from build123d import *

# Parameters (mm, degrees)
F1_DEPTH       = 6.35
F2_R           = 3.81
F3_DEPTH       = 6.35
F5_D           = 2.032
F5_CSINK_D     = 3.175
F5_CSINK_ANGLE = 82
F6_D           = 2.032
F6_CSINK_D     = 3.175
F6_CSINK_ANGLE = 82
F7_SIZE        = 0.508


with BuildPart() as f1:
    # F0 (on Right) → F1 (new body)
    with BuildSketch(Plane.YZ):
        with BuildLine():
            ThreePointArc((-5.08, 12.7), (-3.5921024484, 9.1078975516), (0, 7.62))
            Line((0, 7.62), (0, 12.7))
            Line((0, 12.7), (0, 17.78))
            ThreePointArc((0, 17.78), (-3.5921024484, 16.2921024484), (-5.08, 12.7))
        make_face()
        with BuildLine():
            Line((0, 12.7), (0, 7.62))
            ThreePointArc((0, 7.62), (3.5921024484, 9.1078975516), (5.08, 12.7))
            ThreePointArc((5.08, 12.7), (3.5921024484, 16.2921024484), (0, 17.78))
            Line((0, 17.78), (0, 12.7))
        make_face()
        with BuildLine():
            ThreePointArc((5.08, 12.7), (3.5921024484, 9.1078975516), (0, 7.62))
            ThreePointArc((0, 7.62), (-3.5921024484, 9.1078975516), (-5.08, 12.7))
            Line((-5.08, 12.7), (-5.08, 0))
            ThreePointArc((-5.08, 0), (0, -5.08), (5.08, 0))
            Line((5.08, 0), (5.08, 12.7))
        make_face()
        with BuildLine():
            ThreePointArc((0, 17.78), (3.5921024484, 16.2921024484), (5.08, 12.7))
            Line((5.08, 12.7), (5.08, 32.7368881382))
            Line((5.08, 32.7368881382), (4.2115108686, 31.4493000504))
            ThreePointArc((4.2115108686, 31.4493000504), (2.384915539, 29.8046262283), (0, 29.21))
            Line((0, 29.21), (0, 17.78))
        make_face()
        with BuildLine():
            Line((-5.08, 34.29), (-5.08, 12.7))
            ThreePointArc((-5.08, 12.7), (-3.5921024484, 16.2921024484), (0, 17.78))
            Line((0, 17.78), (0, 29.21))
            ThreePointArc((0, 29.21), (-3.5921024484, 30.6978975516), (-5.08, 34.29))
        make_face()
        with BuildLine():
            Line((4.2115108686, 31.4493000504), (5.08, 32.7368881382))
            Line((5.08, 32.7368881382), (5.08, 34.29))
            ThreePointArc((5.08, 34.29), (4.4853737717, 36.674915539), (2.8406999496, 38.5015108686))
            Line((2.8406999496, 38.5015108686), (0, 34.29))
            Line((0, 34.29), (0, 29.21))
            ThreePointArc((0, 29.21), (2.384915539, 29.8046262283), (4.2115108686, 31.4493000504))
        make_face()
        with BuildLine():
            Line((5.08, 34.29), (5.08, 32.7368881382))
            Line((5.08, 32.7368881382), (26.9371104656, 65.141386999))
            ThreePointArc((26.9371104656, 65.141386999), (25.5662995467, 72.1935978172), (18.5140887285, 70.8227868983))
            Line((18.5140887285, 70.8227868983), (-4.2115108686, 37.1306999496))
            ThreePointArc((-4.2115108686, 37.1306999496), (-0.9693096965, 39.2766660919), (2.8406999496, 38.5015108686))
            ThreePointArc((2.8406999496, 38.5015108686), (4.4853737717, 36.674915539), (5.08, 34.29))
        make_face()
        with BuildLine():
            ThreePointArc((-4.2115108686, 37.1306999496), (-4.8580281603, 35.77524826), (-5.08, 34.29))
            ThreePointArc((-5.08, 34.29), (-3.5921024484, 30.6978975516), (0, 29.21))
            Line((0, 29.21), (0, 34.29))
            Line((0, 34.29), (2.8406999496, 38.5015108686))
            ThreePointArc((2.8406999496, 38.5015108686), (-0.9693096965, 39.2766660919), (-4.2115108686, 37.1306999496))
        make_face()
    extrude(amount=F1_DEPTH)

    # F2 (on face) → F3 (join)
    with BuildSketch(Plane.YZ.offset(6.35)):
        with Locations((0, 12.7)):
            Circle(F2_R)
    extrude(amount=F3_DEPTH)

    # F5 (through all)
    with Locations(Plane.YZ.offset(12.7)):
        with Locations((0, 12.7)):
            CounterSinkHole(F5_D / 2, F5_CSINK_D / 2, counter_sink_angle=F5_CSINK_ANGLE)

    # F6 (through all)
    with Locations(Plane(origin=(0, 0, 0), x_dir=(0, 1, 0), z_dir=(-1, 0, 0))):
        with Locations((0, 0)):
            CounterSinkHole(F6_D / 2, F6_CSINK_D / 2, counter_sink_angle=F6_CSINK_ANGLE)

    # F7
    f7_edges = [f1.edges().sort_by_distance(p)[0] for p in [
        (12.7, -3.81, 12.7),
    ]]
    chamfer(f7_edges, length=F7_SIZE)


solid = f1.part
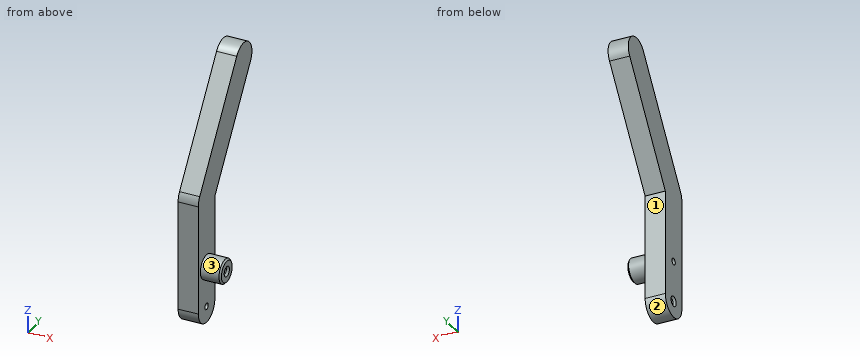
Can you work these out from the model? Positions are in its coordinate system, mm. Face numbers are marked on the shaded views. A direction names the side the tool comes from. Round coordinates to 2 decimals unless told otherwise and drop trailing zeros. Order: outer loops, then holes, each group sorted by start corner. A loop starts at its lowest first (then second) coordinate and runs counter-clockwise, first axis right, second up. Notation, with made-up numbers: (1, 73.25) -> (58, 73.25) arc R21 ccw to (58, 110.25) -> close; hole circle Ø7 at (83, 21). An arc over 180 degrees is marked (long way). Write each question's results on one line, items separated by ' | '. Start each with the question number.
Item 1: Which directions (+Z, -Z, +X, -X, +Y, -Y) give clear straight access to the entire face, cutting with the end or side of a thin tool? Please do the marked faces 1, 2 and 3.
Item 2: If we section it at C-C, the plane y = 0: Write out the boundary of the cut face in (x, z), then the cut area to 3 significant figures.
Item 3: If we section it at A-A, the plane z = 12.7: Write out the boundary of the cut face in (x, y), then the cut area to 3 significant figures.
Item 4: Will these pins go through, and if not, where does the flat tip stop? pin 1 (5 mm diameter, centred on x = 4, z = 13, fed in from +Y); pin 2 (1.5 mm diameter, centred on x = 8, y = 1.5, fed in from +Z); pin 3 (1.2 mm diameter, centred on y = 0, z = 12.7, fed in from +X); pin 4 (6 mm diameter, centred on y = 12.5, z = 50.5, fed in from +X).
Item 5: Please list where these lines run through material, in increasing order: L1, parallel to Z at x = 2.6, y = 0; L2, parallel to Z at x = 7, y = 0; L3, parallel to X at y = -0.5, z = 41.
Item 6: If we section it at D-D, the plane x = 8: Write out the boundary of the cut face in (y, z), then the cut area to 3 significant figures.
Item 7: If we section it at B-B, the plane x = 4: Write out the boundary of the cut face in (y, z).
Results:
1) face 1: -Z, +X, -X, +Y | face 2: -Z, +X, -X | face 3: +X
2) outline: (0, -5.08) -> (6.35, -5.08) -> (6.35, -1.02) -> (0.66, -1.02) -> (0, -1.59) -> close; (0, 1.59) -> (0.66, 1.02) -> (6.35, 1.02) -> (6.35, 8.89) -> (12.19, 8.89) -> (12.7, 9.4) -> (12.7, 11.11) -> (12.04, 11.68) -> (0, 11.68) -> close; (0, 13.72) -> (12.04, 13.72) -> (12.7, 14.29) -> (12.7, 16) -> (12.19, 16.51) -> (6.35, 16.51) -> (6.35, 43.37) -> (0, 43.37) -> close | area: 316 mm2
3) outline: (0, -5.08) -> (6.35, -5.08) -> (6.35, -3.81) -> (12.19, -3.81) -> (12.7, -3.3) -> (12.7, -1.59) -> (12.04, -1.02) -> (0, -1.02) -> close; (0, 1.02) -> (12.04, 1.02) -> (12.7, 1.59) -> (12.7, 3.3) -> (12.19, 3.81) -> (6.35, 3.81) -> (6.35, 5.08) -> (0, 5.08) -> close | area: 86.5 mm2
4) pin 1: stops at y = 5.08 | pin 2: stops at z = 16.44 | pin 3: passes through | pin 4: stops at x = 6.35
5) L1: z = -5.08 to -1.02, 1.02 to 11.68, 13.72 to 43.37 | L2: z = 8.89 to 11.68, 13.72 to 16.51 | L3: x = 0 to 6.35
6) outline: circle Ø7.62 at (0, 12.7); hole circle Ø2.03 at (0, 12.7) | area: 42.4 mm2
7) outline: (-5.08, 0) arc R5.08 ccw to (5.08, 0) -> (5.08, 32.74) -> (26.94, 65.14) arc R5.08 ccw to (18.51, 70.82) -> (-4.21, 37.13) arc R5.08 ccw to (-5.08, 34.29) -> close; hole circle Ø2.03 at (0, 0); hole circle Ø2.03 at (0, 12.7)
